```python
from build123d import *

# Parameters (mm, degrees)
F0_W     = 100
F0_H     = 100
F1_DEPTH = 10
F2_R     = 10
F3_D     = 10


with BuildPart() as f1:
    # F0 (on Top) → F1 (new body)
    with BuildSketch(Plane.XY):
        Rectangle(F0_W, F0_H)
    extrude(amount=F1_DEPTH)

    # F2
    f2_edges = [f1.edges().sort_by_distance(p)[0] for p in [
        (-50, -50, 5),
        (50, -50, 5),
        (50, 50, 5),
        (-50, 50, 5),
    ]]
    fillet(f2_edges, radius=F2_R)

    # F3 (through all)
    with Locations(Plane(origin=(0, 0, 0), x_dir=(1, 0, 0), z_dir=(0, 0, -1))):
        with Locations((0, 0)):
            Hole(F3_D / 2)


solid = f1.part
```
Input: part model. Units: mm. Frame: model coordinates. Give positions to 0.01 mm unless a question says otherwise; leave off trailing zeros. Write each loop counter-clockwise with the first axis right and the second up, starting at its lowest first coordinate (ties: lowest second). Pieces come first, ordered by that corner, then holes. Notation, with made-up numbers: (66, -10) - (118, -10) arc R17 ccw to (118, -1) - close; hole circle Ø5 at (66, 46.25). An arc over 180 degrees is marked (long way). Write item = value, one per line. Start each with the question number.
1. Ray query, L1, parallel to Y at x = 0, z = 7.5; L2, parallel to Y at x = 2, z = 7.5. Return the intervals inside material, ascending.
2. Section query B-B, the plane z = 8.75. Output: boundary loops of the cut face in (x, y).
3. Section query A-A, the plane x = 0. Output: boundary loops of the cut face in (y, z).
4. Mould query, pull axis Y, two halves, no side actions, for faces 1 (the flat face through (-50, -1, 5)), 2 (the cylindrical face through (1.08, 4.88, 5.07)), 3 (the flat face through (-1, -50, 5)). Classes: released by +Y, released by -Y, zero draft, split by the parting line, or undercut.
Check sheet entries:
q1.L1 = -50 to -5, 5 to 50
q1.L2 = -50 to -4.58, 4.58 to 50
q2.outline = (-50, -40) arc R10 ccw to (-40, -50) - (40, -50) arc R10 ccw to (50, -40) - (50, 40) arc R10 ccw to (40, 50) - (-40, 50) arc R10 ccw to (-50, 40) - close; hole circle Ø10 at (0, 0)
q3.outline = (-50, 0) - (-5, 0) - (-5, 10) - (-50, 10) - close; (5, 0) - (50, 0) - (50, 10) - (5, 10) - close
q4.face_1 = zero draft
q4.face_2 = undercut
q4.face_3 = released by -Y
